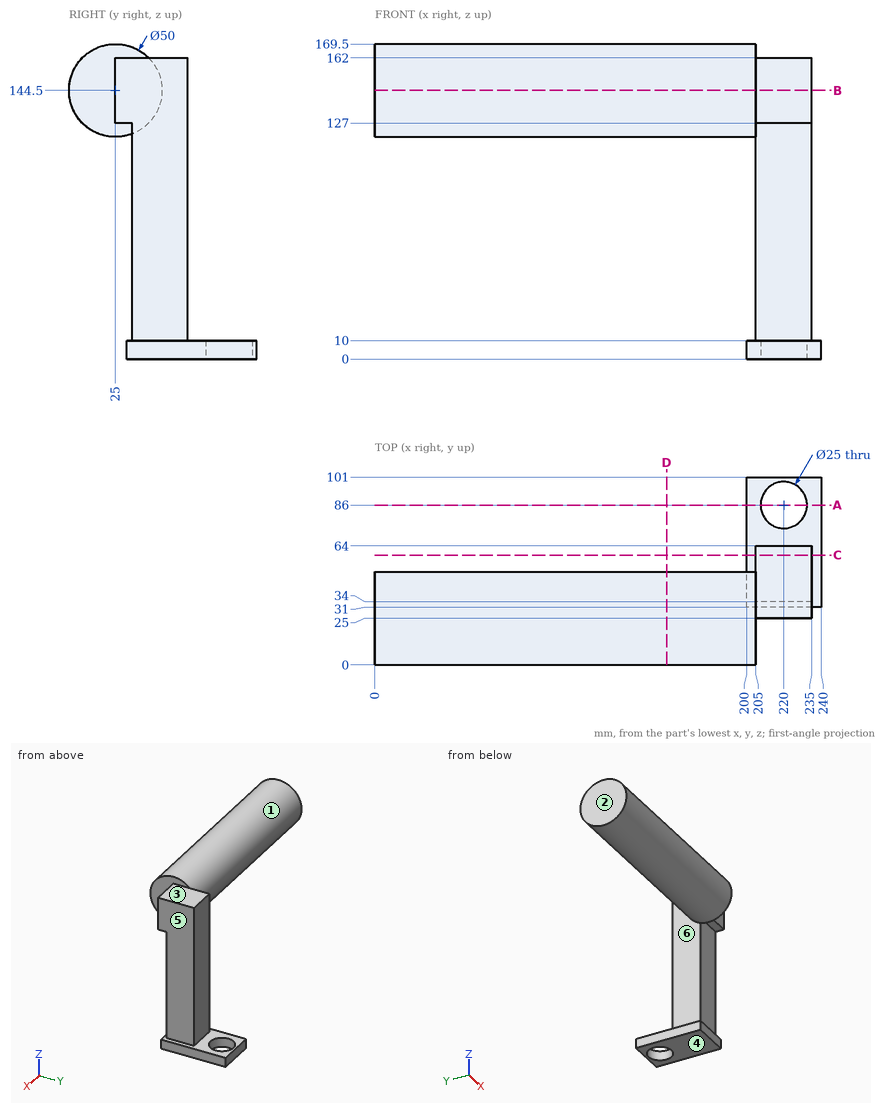
Answer from the drawing. Dimensions are ordinates in mm from the lowest x, y and z of the part. A direction names the side the tool comes from. Coordinates: 2 decimals unless noted, no trailing zeros. Loops run counter-clockwise (first coordinate to the right, second up) from the corner with the lowest first, then second, coordinate; pieces in that order, holes last. Notation, with made-up numbers: (73.5, -34.75) -> (121.5, -34.75) arc R28 cw to (121.5, 1.25) -> close; hole circle Ø1 at (11, -11). An arc over 180 degrees is marked (long way). Answer as CSV lines item,"result".
Q1. The part is cut by section D-D on x = 157. Write down the section's boundary in (y, z).
Findings:
outline,"circle Ø50 at (25, 144.5)"
Q2. Find the intervals of material crossed by probe 1 along Y at (x, z) = (220, 8); probe 2 along Z at (x, y) = (224.5, 44); probe 3 along Y at (x, z) = (221, 76), in increasing order.
Findings:
probe 1,"y = 31 to 73.5, 98.5 to 101"
probe 2,"z = 0 to 162"
probe 3,"y = 34 to 64"
Q3. The part is cut by section B-B on z = 144.5. Write down the section's boundary in (x, y).
Findings:
outline,"(0, 0) -> (205, 0) -> (205, 25) -> (235, 25) -> (235, 64) -> (205, 64) -> (205, 50) -> (0, 50) -> close"
Q4. The part is cut by section C-C on y = 59. Write down the section's boundary in (x, z).
Findings:
outline,"(200, 0) -> (240, 0) -> (240, 10) -> (235, 10) -> (235, 162) -> (205, 162) -> (205, 10) -> (200, 10) -> close"
Q5. For a pull along Z with two mould halves and no side action, classify the marked faces 4, 5 and 6 as +Z half, -Z half, draft (parallel to the pull), parting line (faces both ways), or undercut.
Findings:
face 4,"-Z half"
face 5,"draft"
face 6,"undercut"
Q6. The part is cut by section A-A on y = 86. Write down the section's boundary in (x, z).
Findings:
outline,"(200, 0) -> (207.5, 0) -> (207.5, 10) -> (200, 10) -> close; (232.5, 0) -> (240, 0) -> (240, 10) -> (232.5, 10) -> close"
Q7. A tool of negligible diameter and unlimited length cuts with its end or side. For the marked faces 1, 2 and 3, from which of +Z, -Z, +X, -X, +Y, -Y can it reach the whole face along a straight path? Write none if from no direction.
Findings:
face 1,"-X"
face 2,"+Z, -Z, -X, +Y, -Y"
face 3,"+Z, +X, +Y, -Y"
Q8. Each of these flat-tipped pins is pushed along its axis until it touches: pin 1 (15 mm diameter, centred on x = 215.5, z = 68, fed in from -Y); pin 2 (20 mm diameter, centred on x = 212, y = 61, fed in from +Z); pin 3 (21.5 mm diameter, centred on y = 14.5, z = 143, fed in from +X); pin 4 (7 mm diameter, centred on x = 219.5, y = 29.5, fed in from -Z). Where does it stop, or does it pass through?
Findings:
pin 1,"stops at y = 34"
pin 2,"stops at z = 162"
pin 3,"stops at x = 235"
pin 4,"stops at z = 0"
